The model under review builds one solid part; all positions refer to its coordinate system, in mm. A direction names the side the tool comes from. Round coordinates to 2 decimals unless told otherwise and drop trailing zeros.
Item 1: Machinability: for faces 4 (the face through (-78.745, 21.521, 114.47)), 5 (the face through (-80, 7, 10)), 6 (the face through (-80.44, 28.75, 107.97)), which of the approach directions +Z, -Z, +X, -X, +Y, -Y give a long, thin tool a straight path to every point of the face, cutting with its end or side? Answer none if there is none.
Item 2: Clearance check with flat-ended pins moving along their axes: pin 1 Ø2 at (x, y) = (-79.9, 22) entering from -Z; pin 2 Ø0.8 at (x, y) = (-80, 22.5) entering from +Z. State where each tip first meets the part, or that it passes through.
Item 3: To check wall thickness, follow L1, parallel to Y at x = -79.9, z = 115; L2, parallel to X at y = 22, z = 7; L3, parallel to Z at x = -82, y = 19. State the ranges of each line that lie inside material, in increasing order.
Item 4: Draft analysis for pull direction Y (two halves, no side actions). For faces 1 (the face through (-80, 22, 10)), 2 (the face through (-80, 15, 119.4)), 3 (the face through (-80, 30, 4)), state which applies: +Y half, -Y half, draft (parallel to the pull), parting line (faces both ways), or undercut.
```python
from build123d import *

# Parameters (mm, degrees)
SKETCH_3_W          = 6
SKETCH_3_H          = 30
EXTRUDE_1_DEPTH     = 119.4
SKETCH_4_RX         = 46.310154036
SKETCH_4_RY         = 22.366189945
CUT_EXTRUDE_1_DEPTH = 124.257291874
FILLET_START        = -84
FILLET_1_DEPTH      = 8
SKETCH_5_R          = 1.25
CUT_EXTRUDE_2_DEPTH = 10
CUT_EXTRUDE_START   = -10
SKETCH_6_R          = 1.25
CUT_EXTRUDE_3_DEPTH = 10


with BuildPart() as part:
    # 草图3 → 凸台-拉伸1 (new body)
    with BuildSketch(Plane.XY):
        with Locations((-80.4, 15)):
            Rectangle(SKETCH_3_W, SKETCH_3_H)
    extrude(amount=EXTRUDE_1_DEPTH)

    # 草图4 → 切除-拉伸1 (cut, through all)
    with BuildSketch(Plane.ZY.offset(83.4)):
        with Locations((59.7, 30)):
            Ellipse(SKETCH_4_RX, SKETCH_4_RY)
    extrude(amount=-CUT_EXTRUDE_1_DEPTH, mode=Mode.SUBTRACT)

    # 圆角1: read off the stored shape, not the designer's step
    # 圆角1 outline → 圆角1 (cut)
    with BuildSketch(Plane.YZ.offset(FILLET_START)):
        with BuildLine():
            Line((30, 106.010154036), (30, 112.263898035))
            ThreePointArc((30, 112.263898035), (28.714319891, 107.914425838), (25.270522901, 104.962961112))
            add(Edge.make_bspline(
                [(25.270522901, 104.962961112), (27.608219262, 106.010154036), (30, 106.010154036)],
                knots=[6.05570643, 6.05570643, 6.05570643, 6.283185307, 6.283185307, 6.283185307], degree=2, weights=[0.927453028, 0.957583921, 1]))
        make_face()
        with BuildLine():
            add(Edge.make_bspline(
                [(30, 13.389845964), (27.608219262, 13.389845964), (25.270522901, 14.437038888)],
                knots=[3.141592654, 3.141592654, 3.141592654, 3.369071531, 3.369071531, 3.369071531], degree=2, weights=[1, 0.957583921, 0.927453028]))
            ThreePointArc((25.270522901, 14.437038888), (28.714319891, 11.485574162), (30, 7.136101965))
            Line((30, 7.136101965), (30, 13.389845964))
        make_face()
    extrude(amount=FILLET_1_DEPTH, mode=Mode.SUBTRACT)

    # 草图5 → 切除-拉伸2 (cut)
    with BuildSketch(Plane.XY.offset(119.4)):
        with Locations((-79.9, 22)):
            Circle(SKETCH_5_R)
        with Locations((-79.9, 7)):
            Circle(SKETCH_5_R)
    extrude(amount=-CUT_EXTRUDE_2_DEPTH, mode=Mode.SUBTRACT)

    # 草图6 → 切除-拉伸3 (cut)
    with BuildSketch(Plane(origin=(0, 0, 0), x_dir=(-1, 0, 0), z_dir=(0, 0, -1)).offset(CUT_EXTRUDE_START)):
        with Locations(Location((79.9, 22, 0), (0, 0, 180))):
            Circle(SKETCH_6_R)
        with Locations(Location((79.9, 7, 0), (0, 0, 180))):
            Circle(SKETCH_6_R)
    extrude(amount=CUT_EXTRUDE_3_DEPTH, mode=Mode.SUBTRACT)


solid = part.part
```
Numbers:
1. face 4: +Z
1. face 5: -Z
1. face 6: +X, -X, +Y
2. pin 1: stops at z = 10
2. pin 2: stops at z = 109.4
3. L1: y = 0 to 5.75, 8.25 to 20.75, 23.25 to 30
3. L2: x = -83.4 to -81.15, -78.65 to -77.4
3. L3: z = 0 to 19.38, 100.02 to 119.4
4. face 1: undercut
4. face 2: draft
4. face 3: +Y half
